```python
from build123d import *

# Parameters (mm, degrees)
PAD001_DEPTH    = 2
SKETCH002_R     = 3
SKETCH002_R_2   = 4.9
PAD002_DEPTH    = 8
CHAMFER_SIZE    = 1
CHAMFER001_SIZE = 1
PAD003_DEPTH    = 9
PAD004_DEPTH    = 6
PAD005_DEPTH    = 8.5


with BuildPart() as part:
    # Sketch001 → Pad001 (new body)
    with BuildSketch(Plane.XY):
        with BuildLine():
            Line((-21.73, 22.75), (21.73, 22.75))
            ThreePointArc((22.75, 21.73), (22.451249, 22.451249), (21.73, 22.75))
            Line((22.75, 21.73), (22.75, -15.25))
            ThreePointArc((15.25, -22.75), (20.553301, -20.553301), (22.75, -15.25))
            Line((15.25, -22.75), (-15.25, -22.75))
            ThreePointArc((-22.75, -15.25), (-20.553301, -20.553301), (-15.25, -22.75))
            Line((-22.75, -15.25), (-22.75, 21.73))
            ThreePointArc((-21.73, 22.75), (-22.451249, 22.451249), (-22.75, 21.73))
        make_face()
    extrude(amount=PAD001_DEPTH)

    # Sketch002 → Pad002 (join)
    with BuildSketch(Plane.XY):
        with Locations((-18.05, 18.05)):
            Circle(SKETCH002_R)
        with Locations((18.05, 18.05)):
            Circle(SKETCH002_R)
        with Locations((6.2, -18.15)):
            Circle(SKETCH002_R)
        with Locations((-6.2, -18.15)):
            Circle(SKETCH002_R)
        with Locations((15.8, -16.15)):
            Circle(SKETCH002_R_2)
    extrude(amount=-PAD002_DEPTH)

    # Chamfer
    chamfer_edges = [part.edges().sort_by_distance(p)[0] for p in [
        (15.05, 18.05, -8),
        (-21.05, 18.05, -8),
        (-9.2, -18.15, -8),
        (3.2, -18.15, -8),
        (10.9, -16.15, -8),
    ]]
    chamfer(chamfer_edges, length=CHAMFER_SIZE)

    # Chamfer001
    chamfer001_edges = [part.edges().sort_by_distance(p)[0] for p in [
        (0, -22.75, 2),
    ]]
    chamfer(chamfer001_edges, length=CHAMFER001_SIZE)

    # Sketch003 → Pad003 (join, symmetric)
    with BuildSketch(Plane.XZ.offset(-3)):
        with BuildLine():
            ThreePointArc((-20.8, -0.965685), (-20.677375, -0.349207), (-21.2, 0))
            Line((-21.2, 0), (-15.2, 0))
            ThreePointArc((-15.2, 0), (-16.381381, -0.386204), (-17.106508, -1.395661))
            Line((-19.2, -8), (-17.106508, -1.395661))
            Line((-20.8, -8), (-19.2, -8))
            Line((-21.4, -6.255228), (-20.8, -8))
            Line((-20.8, -5.655228), (-21.4, -6.255228))
            Line((-21.4, -3.910457), (-20.8, -5.655228))
            Line((-20.8, -3.310457), (-21.4, -3.910457))
            Line((-21.4, -1.565685), (-20.8, -3.310457))
            Line((-20.8, -0.965685), (-21.4, -1.565685))
        make_face()
        with BuildLine():
            Line((3, 0), (9, 0))
            ThreePointArc((9, 0), (8.477375, -0.349207), (8.6, -0.965685))
            Line((8.6, -0.965685), (9.2, -1.565685))
            Line((9.2, -1.565685), (8.6, -3.310457))
            Line((8.6, -3.310457), (9.2, -3.910457))
            Line((9.2, -3.910457), (8.6, -5.655228))
            Line((8.6, -5.655228), (9.2, -6.255228))
            Line((9.2, -6.255228), (8.6, -8))
            Line((8.6, -8), (7, -8))
            Line((7, -8), (4.906508, -1.395661))
            ThreePointArc((4.906508, -1.395661), (4.181381, -0.386204), (3, 0))
        make_face()
    extrude(amount=PAD003_DEPTH, both=True)

    # Sketch004 → Pad004 (join, symmetric)
    with BuildSketch(Plane.YZ):
        with BuildLine():
            ThreePointArc((-20.8, -1.023773), (-20.665406, -0.381157), (-21.2, 0))
            Line((-21.2, 0), (-15.2, 0))
            ThreePointArc((-15.2, 0), (-16.381381, -0.386204), (-17.106508, -1.395661))
            Line((-19.2, -8), (-17.106508, -1.395661))
            Line((-20.8, -8), (-19.2, -8))
            Line((-21.4, -6.274591), (-20.8, -8))
            Line((-20.8, -5.674591), (-21.4, -6.274591))
            Line((-21.4, -3.949182), (-20.8, -5.674591))
            Line((-20.8, -3.349182), (-21.4, -3.949182))
            Line((-21.4, -1.623773), (-20.8, -3.349182))
            Line((-20.8, -1.023773), (-21.4, -1.623773))
        make_face()
    extrude(amount=PAD004_DEPTH, both=True)

    # Sketch005 → Pad005 (join, symmetric)
    with BuildSketch(Plane.YZ.offset(-5)):
        with BuildLine():
            Line((15.2, 0), (21.2, 0))
            ThreePointArc((21.2, 0), (20.665406, -0.381157), (20.8, -1.023773))
            Line((20.8, -1.023773), (21.4, -1.623773))
            Line((21.4, -1.623773), (20.8, -3.349182))
            Line((20.8, -3.349182), (21.4, -3.949182))
            Line((21.4, -3.949182), (20.8, -5.674591))
            Line((20.8, -5.674591), (21.4, -6.274591))
            Line((21.4, -6.274591), (20.8, -8))
            Line((20.8, -8), (19.2, -8))
            Line((19.2, -8), (17.106508, -1.395661))
            ThreePointArc((17.106508, -1.395661), (16.381381, -0.386204), (15.2, 0))
        make_face()
    extrude(amount=PAD005_DEPTH, both=True)


solid = part.part
```
Check sheet for the modelled part. Datum: model origin and axes. Units: mm. A direction names the side the tool comes from. Give positions to 0.01 mm unless a question says otherwise; leave off trailing zeros. Write each loop counter-clockwise with the first axis right and the second up, starting at its lowest first coordinate (ties: lowest second). Pieces come first, ordered by that corner, then holes.
Item 1: Scan lines: L1, parallel to X at y = -4, z = -0.5; L2, parallel to Z at x = 8.5, y = -1.5; L3, parallel to Z at x = -13, y = 11. Record each from-to range of solid material in increasing order.
Item 2: Cross-section at A-A (y = 9.5). Enter the section's corners in (x, z).
Item 3: Cross-section at B-B (y = 18.05). Enter the section's corners in (x, z).
Item 4: Gauge pin test, flat ends, axial feed: pin 1 (1 mm diameter, centred on y = -20.5, z = -7.5, fed in from -X); pin 2 (6 mm diameter, centred on x = 13.5, z = -4, fed in from +Y); pin 3 (5 mm diameter, centred on x = 7.5, z = -6, fed in from -Y). Record the tip position at first contact, or that the pin passes through.
Item 5: Access from +Z, -Z, +X, -X, +Y, -Y to the whole of each face (thin tool, end or side, straight path). Record for faces 4 (the face through (0.063, -18.168, -4.744)), 5 (the face through (-20, 3, -8)), 6 (the face through (-4.881, 21.104, -2.474)), 7 (the face through (-16.4, 3.1, -0.4)), 8 (the face through (0.084, -21.104, -2.474)).
Item 6: Draft check along Y on faces 1 (the face through (20.01, -19.91, 1.84)), 2 (the face through (-4.88, 20.67, -0.37)), 3 (the face through (-8.59, -16.34, -3.45)). Enter one of: released by +Y, released by -Y, zero draft, split by the parting line, or undercut.
Report:
1. L1: x = -20.64 to -16.52, 4.32 to 8.44
1. L2: z = -8 to -0.83, -0.3 to 2
1. L3: z = 0 to 2
2. outline: (-22.75, 0) - (-21.2, 0) arc R0.57 cw to (-20.8, -0.97) - (-21.4, -1.57) - (-20.8, -3.31) - (-21.4, -3.91) - (-20.8, -5.66) - (-21.4, -6.26) - (-20.8, -8) - (-19.2, -8) - (-17.11, -1.4) arc R2 cw to (-15.2, 0) - (3, 0) arc R2 cw to (4.91, -1.4) - (7, -8) - (8.6, -8) - (9.2, -6.26) - (8.6, -5.66) - (9.2, -3.91) - (8.6, -3.31) - (9.2, -1.57) - (8.6, -0.97) arc R0.57 cw to (9, 0) - (22.75, 0) - (22.75, 1) - (21.75, 2) - (-21.75, 2) - (-22.75, 1) - close
3. outline: (-22.75, 0) - (-21.05, 0) - (-21.05, -7) - (-20.05, -8) - (-16.05, -8) - (-15.05, -7) - (-15.05, 0) - (-13.5, 0) - (-13.5, -4.37) - (3.5, -4.37) - (3.5, 0) - (15.05, 0) - (15.05, -7) - (16.05, -8) - (20.05, -8) - (21.05, -7) - (21.05, 0) - (22.75, 0) - (22.75, 1) - (21.75, 2) - (-21.75, 2) - (-22.75, 1) - close
4. pin 1: stops at x = -8.25
4. pin 2: stops at y = 20.62
4. pin 3: stops at y = -21.4
5. face 4: -Z
5. face 5: -Z, +X, -X, +Y, -Y
5. face 6: +Y
5. face 7: -Z, -Y
5. face 8: -Y
6. face 1: released by -Y
6. face 2: released by +Y
6. face 3: undercut
